from build123d import *

# Parameters (mm, degrees)
SKETCH_1_W      = 25.4
SKETCH_1_H      = 34
SKETCH_1_R      = 1.6
SKETCH_1_W_2    = 13.4
SKETCH_1_H_2    = 22
EXTRUDE_1_DEPTH = 5
FILLET_1_R      = 2


with BuildPart() as part:
    # 草图1 → 凸台-拉伸1 (new body)
    with BuildSketch(Plane(origin=(0, 0, 0), x_dir=(1, 0, 0), z_dir=(0, 1, 0))):
        Rectangle(SKETCH_1_W, SKETCH_1_H)
        with Locations(Location((-9, 13.5, 0), (0, 0, 270))):
            Circle(SKETCH_1_R, mode=Mode.SUBTRACT)
        with Locations(Location((9, 13.5, 0), (0, 0, 90))):
            Circle(SKETCH_1_R, mode=Mode.SUBTRACT)
        with Locations(Location((9, -13.5, 0), (0, 0, 270))):
            Circle(SKETCH_1_R, mode=Mode.SUBTRACT)
        with Locations(Location((-9, -13.5, 0), (0, 0, 90))):
            Circle(SKETCH_1_R, mode=Mode.SUBTRACT)
        Rectangle(SKETCH_1_W_2, SKETCH_1_H_2, mode=Mode.SUBTRACT)
    extrude(amount=EXTRUDE_1_DEPTH)

    # 圆角1
    fillet_1_edges = [part.edges().sort_by_distance(p)[0] for p in [
        (6.7, 2.5, -11),
        (-6.7, 2.5, -11),
        (-6.7, 2.5, 11),
        (6.7, 2.5, 11),
        (12.7, 2.5, 17),
        (-12.7, 2.5, 17),
        (-12.7, 2.5, -17),
        (12.7, 2.5, -17),
    ]]
    fillet(fillet_1_edges, radius=FILLET_1_R)


solid = part.part
Geometry check sheet. Reference: the model listing, model coordinates, mm. A direction names the side the tool comes from. Give positions to 0.01 mm unless a question says otherwise; leave off trailing zeros. Loops run counter-clockwise (first coordinate to the right, second up) from the corner with the lowest first, then second, coordinate; pieces in that order, holes last. Notation, with made-up numbers: M -28,18 L 12,18 A26 cw 12,36 Z; hole C 31.25,-12 d3. An arc over 180 degrees is marked long. Answer as a JSON object with one key per item and string values. Group by question number.
Item 1: Sectioned sample at C-C on x = -2. Record the boundary of the cut face in (y, z).
Item 2: Gauge pin test, flat end, axial feed: pin 1 (3 mm diameter, centred on x = -9, z = -13.5, fed in from +Y). Record the tip position at first contact, or that the pin passes through.
Item 3: Access from +Z, -Z, +X, -X, +Y, -Y to the whole of each face (thin tool, end or side, straight path). Record for faces 1 (the flat face through (-6.7, 2, 0)), 2 (the cylindrical face through (12.1, 2.54, 16.43)).
Item 4: Material ranges on L1, parallel to X at y = 3.1, z = 13.5; L2, parallel to X at y = 4.45, z = -7; L3, parallel to X at y = 2.85, z = -14, recorded low to high.
Item 5: Sectioned sample at D-D on y = 1.7. Record the boundary of the cut face in (x, z), plus the area to 3 significant figures.
Item 6: Sectioned sample at B-B on x = 9. Record the boundary of the cut face in (y, z), plus the area to 3 significant figures.
Item 7: Sectioned sample at A-A on z = 13.5. Record the boundary of the cut face in (x, y), plus the area to 3 significant figures.
Item 8: Mould release check, pull along X, two halves, no side actions. Record for faces 3 (the cylindrical face through (9.97, 2.46, -12.23)), 4 (the cylindrical face through (-12.13, 2.54, -16.4)), 5 (the cylindrical face through (-8.03, 2.46, 14.77)), 6 (the flat face through (8, 0, 0)): pulls with the +X half, pulls with the -X half, needs draft (parallel to the pull), parting line crosses it, or undercut.
Findings below:
{
 "1": {"outline": "M 0,-17 L 5,-17 L 5,-11 L 0,-11 Z; M 0,11 L 5,11 L 5,17 L 0,17 Z"},
 "2": {"pin 1": "through"},
 "3": {"face 1": "+Y, -Y", "face 2": "+Z, +X, +Y, -Y"},
 "4": {"L1": "-12.7 to -10.6, -7.4 to 7.4, 10.6 to 12.7", "L2": "-12.7 to -6.7, 6.7 to 12.7", "L3": "-12.7 to -10.52, -7.48 to 7.48, 10.52 to 12.7"},
 "5": {"outline": "M -12.7,-15 A2 ccw -10.7,-17 L 10.7,-17 A2 ccw 12.7,-15 L 12.7,15 A2 ccw 10.7,17 L -10.7,17 A2 ccw -12.7,15 Z; hole C -9,-13.5 d3.2; hole C -9,13.5 d3.2; hole M -6.7,-9 A2 ccw -4.7,-11 L 4.7,-11 A2 ccw 6.7,-9 L 6.7,9 A2 ccw 4.7,11 L -4.7,11 A2 ccw -6.7,9 Z; hole C 9,-13.5 d3.2; hole C 9,13.5 d3.2", "area": "537 mm2"},
 "6": {"outline": "M 0,-17 L 5,-17 L 5,-15.1 L 0,-15.1 Z; M 0,-11.9 L 5,-11.9 L 5,11.9 L 0,11.9 Z; M 0,15.1 L 5,15.1 L 5,17 L 0,17 Z", "area": "138 mm2"},
 "7": {"outline": "M -12.7,0 L -10.6,0 L -10.6,5 L -12.7,5 Z; M -7.4,0 L 7.4,0 L 7.4,5 L -7.4,5 Z; M 10.6,0 L 12.7,0 L 12.7,5 L 10.6,5 Z", "area": "95.0 mm2"},
 "8": {"face 3": "undercut", "face 4": "pulls with the -X half", "face 5": "undercut", "face 6": "needs draft"}
}
